```python
from build123d import *

# Parameters (mm, degrees)
SKETCH1_W           = 115
SKETCH1_H           = 210
BOSS_EXTRUDE1_DEPTH = 30
SKETCH3_W           = 60
SKETCH3_H           = 60
BOSS_EXTRUDE2_DEPTH = 50
SKETCH4_R           = 15
BOSS_EXTRUDE3_DEPTH = 50
FILLET1_R           = 10
SKETCH7_W           = 45
SKETCH7_H           = 8
BOSS_EXTRUDE6_DEPTH = 80
CUT_EXTRUDE1_DEPTH  = 226


with BuildPart() as part:
    # Sketch1 → Boss-Extrude1 (new body)
    with BuildSketch(Plane.XY):
        Rectangle(SKETCH1_W, SKETCH1_H)
    extrude(amount=BOSS_EXTRUDE1_DEPTH)

    # Sketch3 → Boss-Extrude2 (add, symmetric)
    with BuildSketch(Plane(origin=(0, 0, 0), x_dir=(1, 0, 0), z_dir=(0, 1, 0))):
        with Locations((0, 30)):
            Rectangle(SKETCH3_W, SKETCH3_H)
    extrude(amount=BOSS_EXTRUDE2_DEPTH, both=True)

    # Sketch4 → Boss-Extrude3 (add, symmetric)
    with BuildSketch(Plane(origin=(0, 0, 0), x_dir=(1, 0, 0), z_dir=(0, 1, 0))):
        with BuildLine():
            Line((-40, 272.819293264), (-40, 57.180706736))
            ThreePointArc((-40, 57.180706736), (0, 50), (40, 57.180706736))
            Line((40, 57.180706736), (40, 272.819293264))
            ThreePointArc((40, 272.819293264), (0, 280), (-40, 272.819293264))
        make_face()
        with Locations(Location((0, 240, 0), (0, 0, 270))):
            Circle(SKETCH4_R, mode=Mode.SUBTRACT)
        with Locations(Location((0, 90, 0), (0, 0, 270))):
            Circle(SKETCH4_R, mode=Mode.SUBTRACT)
    extrude(amount=BOSS_EXTRUDE3_DEPTH, both=True)

    # Fillet1
    fillet1_edges = [part.edges().sort_by_distance(p)[0] for p in [
        (0, -50, 0),
        (-30, 0, 0),
        (30, 0, 0),
        (0, 50, 0),
    ]]
    fillet(fillet1_edges, radius=FILLET1_R)

    # Sketch7 → Boss-Extrude6 (add)
    with BuildSketch(Plane.ZY.offset(40)):
        with Locations((-165, 54)):
            Rectangle(SKETCH7_W, SKETCH7_H)
    extrude(amount=-BOSS_EXTRUDE6_DEPTH)

    # Sketch11 → Cut-Extrude1 (cut)
    with BuildSketch(Plane.ZY.offset(40)):
        with BuildLine():
            Line((-205, 10), (-205, -50))
            Line((-205, -50), (-125, -50))
            Line((-125, -50), (-125, 10))
            ThreePointArc((-125, 10), (-165, 50), (-205, 10))
        make_face()
    extrude(amount=-CUT_EXTRUDE1_DEPTH, mode=Mode.SUBTRACT)


solid = part.part
```
Here's how the part is built. I have some questions about the finished solid (model axes, mm). A direction names the side the tool comes from. Give positions to 0.01 mm unless a question says otherwise; leave off trailing zeros. Order: outer loops, then holes, each group sorted by start corner. A loop starts at its lowest first (then second) coordinate and runs counter-clockwise, first axis right, second up. Notation, with made-up numbers: M 5,13 L 34,13 A20 ccw 34,43 Z; hole C 58.25,45 d3. An arc over 180 degrees is marked long. Use a Markdown table: item, result. Add a question column.
1. I need wall thicknesses on probe 1 along X at (y, z) = (19, -90); probe 2 along Z at (x, y) = (-39.5, -35); probe 3 along Z at (x, y) = (50, 50). Which ranges of each line are inside material? Lowest first, please. Write a range as from..to.
2. Suppose I cut it at B-B (x = 0). List the corners of the cut face in (y, z) for me.
3. If we mould it in two halves opening along X, with no side actions, what happens to faces 1 (the flat face through (30, 1, -32)), 2 (the flat face through (-1, 50, -224)), 3 (the cylindrical face through (4.506, -0.7, -225.693))? For each: +X half, -X half, draft (parallel to the pull), parting line (faces both ways), or undercut.
4. On a 3-axis mill with a long thin cutter (end or side, diameter ignored), from which of +Z, -Z, +X, -X, +Y, -Y can I reach the whole of each face in a straight line? I mean faces 4 (the flat face through (-9, 50, -77)), 5 (the cylindrical face through (-32.85, 0.84, -3.01)), 6 (the flat face through (40, 5, -211)), 7 (the flat face through (-1, -20, -125)), 8 (the flat face through (-1, -50, -68)). Say none if no direction works.
5. Suppose I cut it at A-A (y = 32). List the corners of the cut face in (x, z) for me, and give its area (3 significant figures).
6. For pin 1 Ø2.5 at (x, y) = (20, 55.5) entering from -Z; pin 2 Ø13 at (y, z) = (-18.5, -23) entering from -X; pin 3 Ø24 at (x, z) = (16.5, -107.5) entering from +Y, each with a flat end and sliding along its axis, tell me the tip position at first contact or that it passes through.
7. Suppose I cut it at C-C (z = -90). List the corners of the cut face in (x, y) for me, and give its area (3 significant figures).
8. Suppose I cut it at D-D (x = -33.5). List the corners of the cut face in (y, z) for me.
Results list:
| question | item | result |
|---|---|---|
| 1 | probe 1 | x = -40..-15, 15..40 |
| 1 | probe 2 | z = -273..-205, -125..-57, -0.01..30 |
| 1 | probe 3 | z = 0..30 |
| 2 | outline | M -105,0 L -60,0 A10 cw -50,-10 L -50,-75 L 50,-75 L 50,-10 A10 cw 60,0 L 105,0 L 105,30 L -105,30 Z; M -50,-280 L 50,-280 L 50,-255 L -50,-255 Z; M -50,-225 L 50,-225 L 50,-187.5 L 58,-187.5 L 58,-142.5 L 50,-142.5 L 50,-105 L -50,-105 L -50,-125 L 10,-125 A40 cw 10,-205 L -50,-205 Z |
| 3 | face 1 | +X half |
| 3 | face 2 | draft |
| 3 | face 3 | undercut |
| 4 | face 4 | +X, -X, +Y |
| 4 | face 5 | -X, +Y, -Y |
| 4 | face 6 | -Z, +X, +Y, -Y |
| 4 | face 7 | +X, -X, -Y |
| 4 | face 8 | -Z, +X, -X, -Y |
| 5 | outline | M -57.5,0 L -40,0 A10 cw -30,-10 L -30,-53.98 A115 ccw -40,-57.18 L -40,-131.59 L 40,-131.59 L 40,-57.18 A115 ccw 30,-53.98 L 30,-10 A10 cw 40,0 L 57.5,0 L 57.5,30 L -57.5,30 Z; M -40,-272.82 A115 ccw 40,-272.82 L 40,-198.41 L -40,-198.41 Z; hole C 0,-240 d30; hole C 0,-90 d30 |
| 5 | area | 17,800 mm² |
| 6 | pin 1 | stops at z = -187.5 |
| 6 | pin 2 | stops at x = -30 |
| 6 | pin 3 | stops at y = 50 |
| 7 | outline | M -40,-50 L -15,-50 L -15,50 L -40,50 Z; M 15,-50 L 40,-50 L 40,50 L 15,50 Z |
| 7 | area | 5,000 mm² |
| 8 | outline | M -105,0 L -60,0 A10 cw -53.5,-2.4 L 53.5,-2.4 A10 cw 60,0 L 105,0 L 105,30 L -105,30 Z; M -50,-275.01 L 50,-275.01 L 50,-187.5 L 58,-187.5 L 58,-142.5 L 50,-142.5 L 50,-54.99 L -50,-54.99 L -50,-125 L 10,-125 A40 cw 10,-205 L -50,-205 Z |
